Autodesk Inventor part; units mm, degrees
ref_plane "YZ Plane" through (0, 0, 0) normal (1, 0, 0) x (0, 1, 0)
ref_plane "XZ Plane" through (0, 0, 0) normal (0, 1, 0) x (-1, 0, 0)
ref_plane "XY Plane" through (0, 0, 0) normal (0, 0, 1) x (1, 0, 0)
sketch "Sketch1" plane through (0, 0, 0) normal (0, 1, 0) x (-1, 0, 0)
  line L0 (-47.4268, -17.2867) -> (-59.4268, -17.2867)
  line L1 (-59.4268, -17.2867) -> (-59.4268, 282.7133)
  line L2 (-59.4268, 282.7133) -> (-47.4268, 282.7133)
  line L3 (-47.4268, 282.7133) -> (-47.4268, -17.2867)
  point P0 (0, 0)
  dimension "d0" = 300
  dimension "d1" = 12
extrude "Extrusion1" add sketch "Sketch1" along normal blind 8
sketch "Sketch2" plane through (0, 8, 0) normal (0, 1, 0) x (1, 0, 0)
  circle A0 centre (53.4268, -270.2133) radius 1.75
  line L0 (59.4268, -282.7133) -> (59.4268, 17.2867)
  line L1 (47.4268, -282.7133) -> (59.4268, -282.7133)
  circle A1 centre (53.4268, -245.2133) radius 1.75
  circle A2 centre (53.4268, -220.2133) radius 1.75
  circle A3 centre (53.4268, -195.2133) radius 1.75
  circle A4 centre (53.4268, -170.2133) radius 1.75
  circle A5 centre (53.4268, -145.2133) radius 1.75
  circle A6 centre (53.4268, -120.2133) radius 1.75
  circle A7 centre (53.4268, -95.2133) radius 1.75
  circle A8 centre (53.4268, -70.2133) radius 1.75
  circle A9 centre (53.4268, -45.2133) radius 1.75
  point P0 (0, 0)
  dimension "d4" = 3.5
  dimension "d5" = 6
  dimension "d6" = 12.5
  dimension "d9" = 25
extrude "Extrusion2" cut sketch "Sketch2" against normal through all
properties part number "MGN12H_rail" material "Stainless Steel"
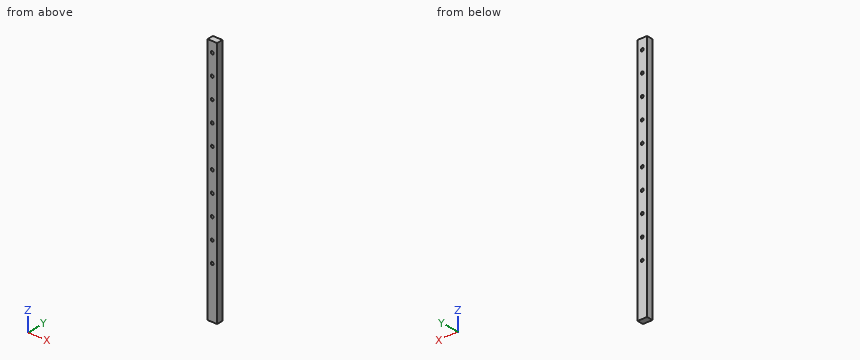
The listing builds one solid part. Answer for the finished solid, in the listing's coordinates (mm). Give positions to 0.01 mm unless a question says otherwise; leave off trailing zeros.
1) Find section A-A on y = 4. Give the number of separate pieces and of enclosed holes in the cut face, then the cut area to 3 significant figures.
Reported:
separate pieces: 1
enclosed holes: 10
area: 3,500 mm2
2) Given P1, Ø2, axis at x = 53.43, z = 145.21, coming from the -Y side, flat-ended and moving along its own axis, determine where the tip first touches the part or whether it passes through.
Reported:
P1: passes through
3) Consider line 1 along X through (y, z) = (3, 220); line 2 along X through (y, z) = (3.25, 246.5). Determine where each line is inside the solid, lowest interval first.
Reported:
line 1: x = 47.43 to 51.69, 55.16 to 59.43
line 2: x = 47.43 to 52.24, 54.61 to 59.43
